Build history of the part. All positions in model axes, mm. Face numbers are marked on the shaded views. A direction names the side the tool comes from. Give positions to 0.01 mm unless a question says otherwise; leave off trailing zeros. Order: outer loops, then holes, each group sorted by start corner. A loop starts at its lowest first (then second) coordinate and runs counter-clockwise, first axis right, second up. Notation, with made-up numbers: (-23.75, 22) - (-14.75, 22) arc R9 ccw to (-14.75, 38) - close; hole circle Ø4 at (67, 7). An arc over 180 degrees is marked (long way). One line per item, written item: value.
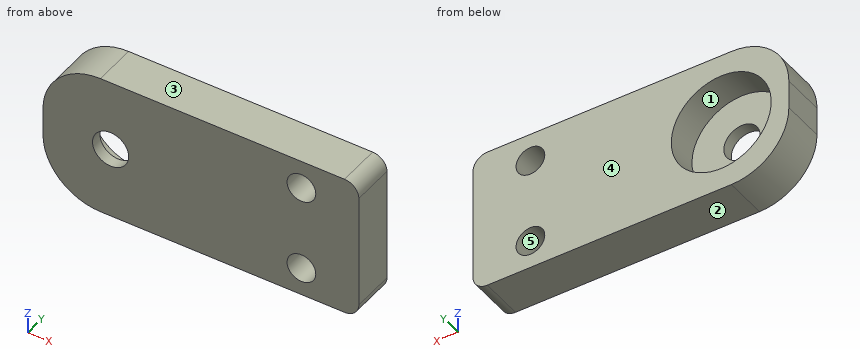
```python
from build123d import *

# Parameters (mm, degrees)
SKETCH1_W           = 69.85
SKETCH1_H           = 31.75
SKETCH1_R           = 4
SKETCH1_R_2         = 3.175
BOSS_EXTRUDE1_DEPTH = 9.525
SKETCH2_R           = 11.05
CUT_EXTRUDE1_DEPTH  = 7
FILLET2_R           = 12.7
FILLET3_R           = 3.175


with BuildPart() as part:
    # Sketch1 → Boss-Extrude1 (new body)
    with BuildSketch(Plane(origin=(0, 0, 0), x_dir=(1, 0, 0), z_dir=(0, 1, 0))):
        with Locations((34.925, 15.875)):
            Rectangle(SKETCH1_W, SKETCH1_H)
        with Locations(Location((14.950000072, 15.875, 0), (0, 0, 90))):
            Circle(SKETCH1_R, mode=Mode.SUBTRACT)
        with Locations(Location((57.15, 25.441087639, 0), (0, 0, 90))):
            Circle(SKETCH1_R_2, mode=Mode.SUBTRACT)
        with Locations(Location((57.15, 6.308912361, 0), (0, 0, 90))):
            Circle(SKETCH1_R_2, mode=Mode.SUBTRACT)
    extrude(amount=BOSS_EXTRUDE1_DEPTH)

    # Sketch2 → Cut-Extrude1 (cut)
    with BuildSketch(Plane(origin=(0, 9.525, 0), x_dir=(1, 0, 0), z_dir=(0, 1, 0))):
        with Locations(Location((14.950000072, 15.875, 0), (0, 0, 270))):
            Circle(SKETCH2_R)
    extrude(amount=-CUT_EXTRUDE1_DEPTH, mode=Mode.SUBTRACT)

    # Fillet2
    fillet2_edges = [part.edges().sort_by_distance(p)[0] for p in [
        (0, 4.7625, -31.75),
        (0, 4.7625, 0),
    ]]
    fillet(fillet2_edges, radius=FILLET2_R)

    # Fillet3
    fillet3_edges = [part.edges().sort_by_distance(p)[0] for p in [
        (69.85, 4.7625, -31.75),
        (69.85, 4.7625, 0),
    ]]
    fillet(fillet3_edges, radius=FILLET3_R)


solid = part.part
```
(1) Slice it at B-B, the plane z = -24. Give the cut face in (x, y) (3 decimals), and give its area (3 significant figures).
Completed:
outline: (1.004, 0) - (54.321, 0) - (54.321, 9.525) - (22.439, 9.525) - (22.439, 2.525) - (7.461, 2.525) - (7.461, 9.525) - (1.004, 9.525) - close; (59.979, 0) - (69.85, 0) - (69.85, 9.525) - (59.979, 9.525) - close
area: 497 mm²
(2) Slice it at A-A, the plane x = 57.15. Give the cut face in (y, z) (3 decimals), and give its area (3 significant figures).
Completed:
outline: (0, -31.75) - (9.525, -31.75) - (9.525, -28.616) - (0, -28.616) - close; (0, -22.266) - (9.525, -22.266) - (9.525, -9.484) - (0, -9.484) - close; (0, -3.134) - (9.525, -3.134) - (9.525, 0) - (0, 0) - close
area: 181 mm²
(3) 3-axis set-ups, long thin cutter, end or side, ignore diameter. For the marked faces 1 and 2: which of +Z, -Z, +X, -X, +Y, -Y reach the whole face in a straight line?
Completed:
face 1: +Y
face 2: -Z, +X, -X, +Y, -Y
(4) Drill centre lines: line 1 (Z direction, x = 57.15, y = 6.5); line 2 (Z direction, x = 59, y = 3.25); line 3 (X direction, y = 3.25, z = -24). Where is each one in solid material? Low to high.
Completed:
line 1: -31.75 to -28.62, -22.27 to -9.48, -3.13 to 0
line 2: -31.75 to -28.02, -22.86 to -8.89, -3.73 to 0
line 3: 1 to 7.46, 22.44 to 54.32, 59.98 to 69.85
(5) Pull direction Z, two halves, no side cores. Call the marked faces 3, 4 and 5: +Z half, -Z half, draft (parallel to the pull), parting line (faces both ways), or undercut.
Completed:
face 3: +Z half
face 4: draft
face 5: undercut
(6) Pin check, flat tips, straight feed: P1, Ø10.5, axis at x = 14.95, z = -15.875, coming from the +Y side (3 decimals); P2, Ø4, axis at y = 1, z = -7.5, coming from the -X side. Stop position of each tip, or through.
Completed:
P1: y = 2.525
P2: x = 0.41
(7) Slice it at C-C, the plane y = 3.75. Give the cut face in (x, z) (3 decimals).
Completed:
outline: (0, -19.05) arc R12.7 ccw to (12.7, -31.75) - (66.675, -31.75) arc R3.175 ccw to (69.85, -28.575) - (69.85, -3.175) arc R3.175 ccw to (66.675, 0) - (12.7, 0) arc R12.7 ccw to (0, -12.7) - close; hole circle Ø22.1 at (14.95, -15.875); hole circle Ø6.35 at (57.15, -25.441); hole circle Ø6.35 at (57.15, -6.309)
(8) Slice it at D-D, the plane x = 10. Give the cut face in (y, z) (3 decimals).
Completed:
outline: (0, -31.46) - (9.525, -31.46) - (9.525, -25.754) - (2.525, -25.754) - (2.525, -5.996) - (9.525, -5.996) - (9.525, -0.29) - (0, -0.29) - close
